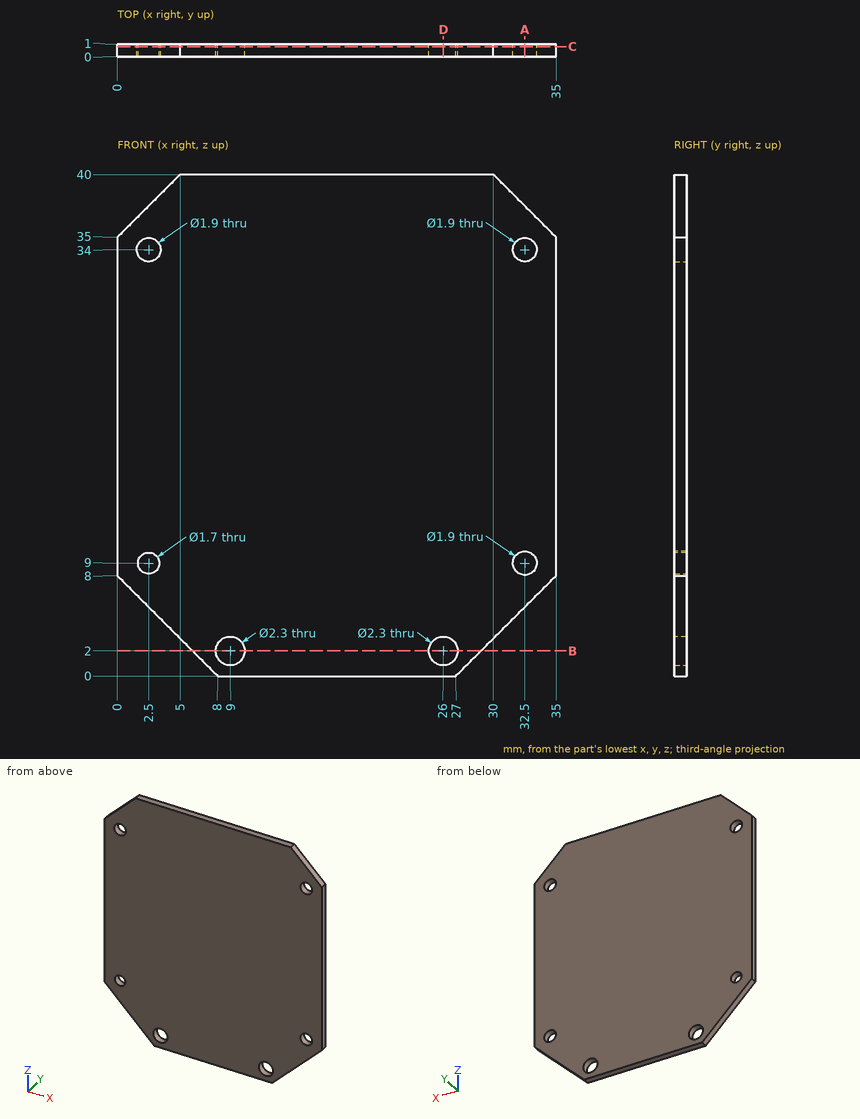
Drawing for the job (mm, zero at the part's lowest x, y, z). Round coordinates to 2 decimals unless told otherwise and drop trailing zeros. Loops run counter-clockwise (first coordinate to the right, second up) from the corner with the lowest first, then second, coordinate; pieces in that order, holes last. Notation, with made-up numbers: (-34, 83) -> (-11, 83) arc R24 ccw to (-11, 94) -> close; hole circle Ø5 at (24.25, 20.25). An arc over 180 degrees is marked (long way). Answer as CSV lines item,"result". Start each with the question number.
1) Probe line 1 along X through (y, z) = (0.6, 9); line 2 along X through (y, z) = (0.55, 34); line 3 along Z through (x, y) = (33, 0.25). List the from-to ranges inside material, lowest first.
2) Slice it at D-D (x = 26). List the corners of the cut face in (y, z), plus the area to 3 significant figures.
3) Slice it at B-B (z = 2). List the corners of the cut face in (x, y), plus the area to 3 significant figures.
4) Slice it at A-A (x = 32.5). List the corners of the cut face in (y, z).
5) Slice it at C-C (y = 0.8). List the corners of the cut face in (x, z), plus the area to 3 significant figures.
Filled in:
1,line 1,"x = 0 to 1.65, 3.35 to 31.55, 33.45 to 35"
1,line 2,"x = 0 to 1.55, 3.45 to 31.55, 33.45 to 35"
1,line 3,"z = 6 to 8.19, 9.81 to 33.19, 34.81 to 37"
2,outline,"(0, 0) -> (1, 0) -> (1, 0.85) -> (0, 0.85) -> close; (0, 3.15) -> (1, 3.15) -> (1, 40) -> (0, 40) -> close"
2,area,"37.7 mm2"
3,outline,"(6, 0) -> (7.85, 0) -> (7.85, 1) -> (6, 1) -> close; (10.15, 0) -> (24.85, 0) -> (24.85, 1) -> (10.15, 1) -> close; (27.15, 0) -> (29, 0) -> (29, 1) -> (27.15, 1) -> close"
3,area,"18.4 mm2"
4,outline,"(0, 5.5) -> (1, 5.5) -> (1, 8.05) -> (0, 8.05) -> close; (0, 9.95) -> (1, 9.95) -> (1, 33.05) -> (0, 33.05) -> close; (0, 34.95) -> (1, 34.95) -> (1, 37.5) -> (0, 37.5) -> close"
5,outline,"(0, 8) -> (8, 0) -> (27, 0) -> (35, 8) -> (35, 35) -> (30, 40) -> (5, 40) -> (0, 35) -> close; hole circle Ø1.9 at (2.5, 34); hole circle Ø1.7 at (2.5, 9); hole circle Ø2.3 at (9, 2); hole circle Ø2.3 at (26, 2); hole circle Ø1.9 at (32.5, 9); hole circle Ø1.9 at (32.5, 34)"
5,area,"1,290 mm2"
